For this review, take the finished solid that the model builds, in its own axes (mm). A direction names the side the tool comes from. Give positions to 0.01 mm unless a question says otherwise; leave off trailing zeros. Write each loop counter-clockwise with the first axis right and the second up, starting at its lowest first coordinate (ties: lowest second). Pieces come first, ordered by that corner, then holes. Notation, with made-up numbers: (-14.75, 56.5) -> (17.25, 56.5) arc R20 ccw to (17.25, 81.5) -> close; hole circle Ø7 at (-19.5, 22.5). An arc over 180 degrees is marked (long way). Write item = value, one per line.
```python
from build123d import *

# Parameters (mm, degrees)
SKETCH1_W           = 306.999208532
SKETCH1_H           = 400
SKETCH1_W_2         = 113.639208532
SKETCH1_H_2         = 50
BOSS_EXTRUDE1_DEPTH = 9
SKETCH2_W           = 95
SKETCH2_H           = 300
CUT_EXTRUDE1_DEPTH  = 460.151907085
SKETCH3_W           = 40
SKETCH3_H           = 15
CUT_EXTRUDE2_DEPTH  = 10
SKETCH4_W           = 10
SKETCH4_H           = 20
CUT_EXTRUDE3_DEPTH  = 100


with BuildPart() as part:
    # Sketch1 → Boss-Extrude1 (new body)
    with BuildSketch(Plane.XY):
        with Locations((-170.312553906, 125.4)):
            Rectangle(SKETCH1_W, SKETCH1_H)
        with Locations((-251.992553906, 283.4)):
            Rectangle(SKETCH1_W_2, SKETCH1_H_2, mode=Mode.SUBTRACT)
        with Locations((-251.992553906, -32.6)):
            Rectangle(SKETCH1_W_2, SKETCH1_H_2, mode=Mode.SUBTRACT)
    extrude(amount=BOSS_EXTRUDE1_DEPTH)

    # Sketch2 → Cut-Extrude1 (cut, through all)
    with BuildSketch(Plane(origin=(0, 0, 0), x_dir=(-1, 0, 0), z_dir=(0, 0, -1))):
        with Locations((64.31294964, 125.4)):
            Rectangle(SKETCH2_W, SKETCH2_H)
    extrude(amount=-CUT_EXTRUDE1_DEPTH, mode=Mode.SUBTRACT)

    # Sketch3 → Cut-Extrude2 (cut)
    with BuildSketch(Plane(origin=(0, 0, 0), x_dir=(-1, 0, 0), z_dir=(0, 0, -1))):
        with Locations((91.81294964, 282.9)):
            Rectangle(SKETCH3_W, SKETCH3_H)
    extrude(amount=-CUT_EXTRUDE2_DEPTH, mode=Mode.SUBTRACT)

    # Sketch4 → Cut-Extrude3 (cut)
    with BuildSketch(Plane(origin=(0, 0, 0), x_dir=(-1, 0, 0), z_dir=(0, 0, -1))):
        with Locations((116.81294964, 280.4)):
            Rectangle(SKETCH4_W, SKETCH4_H)
    extrude(amount=-CUT_EXTRUDE3_DEPTH, mode=Mode.SUBTRACT)


solid = part.part
```
(1) Take a section at D-D (y = 2). Write out the cut boundary in (x, z), plus the area to 3 significant figures.
Answers below:
outline = (-323.81, 0) -> (-111.81, 0) -> (-111.81, 9) -> (-323.81, 9) -> close
area = 1,910 mm^2
(2) Tool access review of faces 5 (the face through (-71.813, 283, 4)), 6 (the face through (-64, -24.6, 4)), 7 (the face through (-16.813, 300, 4)): name each direction out of +Z, -Z, +X, -X, +Y, -Y from which nothing blocks a thin tool from reaching the whole face with its end or side.
Answers below:
face_5 = +Z, -Z
face_6 = +Z, -Z, +X
face_7 = +Z, -Z, +X, +Y, -Y
(3) Take a section at C-C (z = 3.5). Write out the cut boundary in (x, y).
Answers below:
outline = (-323.81, -74.6) -> (-16.81, -74.6) -> (-16.81, -24.6) -> (-111.81, -24.6) -> (-111.81, 270.4) -> (-121.81, 270.4) -> (-121.81, 290.4) -> (-71.81, 290.4) -> (-71.81, 275.4) -> (-16.81, 275.4) -> (-16.81, 325.4) -> (-323.81, 325.4) -> close; hole (-308.81, -57.6) -> (-195.17, -57.6) -> (-195.17, -7.6) -> (-308.81, -7.6) -> close; hole (-308.81, 258.4) -> (-195.17, 258.4) -> (-195.17, 308.4) -> (-308.81, 308.4) -> close
(4) The part is to be moulded in two halves that separate along Y. For faces 1 (the face through (-44, 275.4, 4)), 2 (the face through (-207, 128, 0)), 3 (the face through (-172, 325.4, 4)), 4 (the face through (-253, -57.6, 4)), say which applies: released by +Y, released by -Y, zero draft, split by the parting line, or undercut.
Answers below:
face_1 = undercut
face_2 = zero draft
face_3 = released by +Y
face_4 = undercut
(5) Take a section at B-B (x = -227.5). Write out the cut boundary in (y, z).
Answers below:
outline = (-74.6, 0) -> (-57.6, 0) -> (-57.6, 9) -> (-74.6, 9) -> close; (-7.6, 0) -> (258.4, 0) -> (258.4, 9) -> (-7.6, 9) -> close; (308.4, 0) -> (325.4, 0) -> (325.4, 9) -> (308.4, 9) -> close
(6) Take a section at A-A (y = 299). Write out the cut boundary in (x, z), plus the area to 3 significant figures.
Answers below:
outline = (-323.81, 0) -> (-308.81, 0) -> (-308.81, 9) -> (-323.81, 9) -> close; (-195.17, 0) -> (-16.81, 0) -> (-16.81, 9) -> (-195.17, 9) -> close
area = 1,740 mm^2
(7) To check wall thickness, follow probe 1 along Y at (x, z) = (-299, 4.25); probe 2 along X at (y, z) = (-21, 4.5); probe 3 along X at (y, z) = (-26.5, 6.25). State the ranges of each line that lie inside material, in increasing order.
Answers below:
probe_1 = -74.6 to -57.6, -7.6 to 258.4, 308.4 to 325.4
probe_2 = -323.81 to -308.81, -195.17 to -111.81
probe_3 = -323.81 to -308.81, -195.17 to -16.81
(8) For pin 1 (4 mm diameter, centred on y = -15.5, z = 6, fed in from +X), flat-tipped, find the tip position at first contact; note if it passes through.
Answers below:
pin_1 = -111.81
